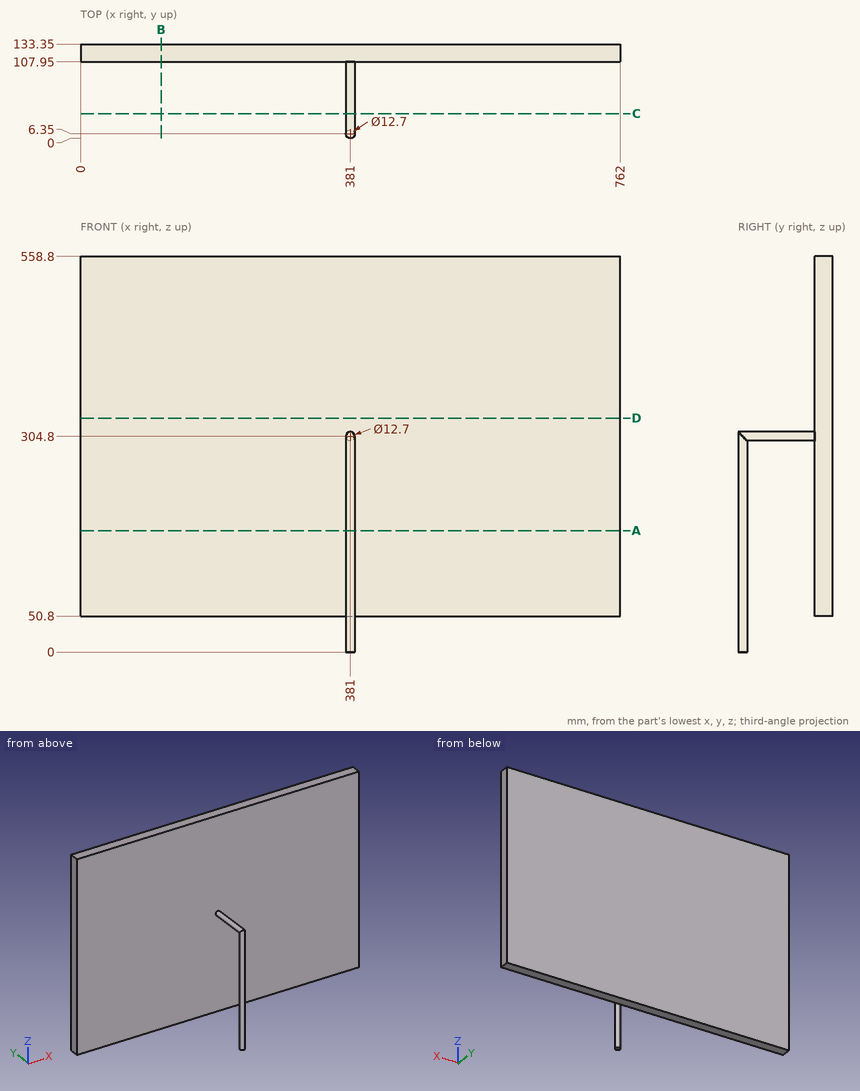
Here's the drawing with two shaded views (mm, measured from the low corner). I have some questions. Give positions to 0.01 mm unless a question says otherwise; leave off trailing zeros. Write each loop counter-clockwise with the first axis right and the second up, starting at its lowest first coordinate (ties: lowest second). Pieces come first, ordered by that corner, then holes. Notation, with made-up numbers: (58.5, 88) -> (84.5, 88) arc R26 cw to (84.5, 114) -> close; hole circle Ø3 at (-2.75, -6.5). An arc over 180 degrees is marked (long way). Use one line per item in the form item = value. Start each with the question number.
1. Imagine slicing it at B-B on x = 114. List the corners of the cut face in (y, z) for me, plus the area to 3 significant figures.
2. Imagine slicing it at D-D on z = 330.5. List the corners of the cut face in (x, y) for me, plus the area to 3 significant figures.
3. Imagine slicing it at C-C on y = 35. List the corners of the cut face in (x, z) for me, plus the area to 3 significant figures.
4. If I drill on L1, parallel to Y at x = 698, z = 111.5; L2, parallel to Z at x = 264.5, y = 117.5, over which ranges is the centre line in solid material (lowest first)?
5. Imagine slicing it at A-A on z = 171.5. List the corners of the cut face in (x, y) for me.
6. Will this pin go through, and if not, where does the flat tip stop? pin 1 Ø10 at (x, z) = (165, 288) entering from -Y.
Entries:
q1.outline = (107.95, 50.8) -> (133.35, 50.8) -> (133.35, 558.8) -> (107.95, 558.8) -> close
q1.area = 12,900 mm²
q2.outline = (0, 107.95) -> (762, 107.95) -> (762, 133.35) -> (0, 133.35) -> close
q2.area = 19,400 mm²
q3.outline = circle Ø12.7 at (381, 304.8)
q3.area = 127 mm²
q4.L1 = 107.95 to 133.35
q4.L2 = 50.8 to 558.8
q5.outline = (0, 107.95) -> (762, 107.95) -> (762, 133.35) -> (0, 133.35) -> close; circle Ø12.7 at (381, 6.35)
q6.pin_1 = 107.95
